```python
from build123d import *

# Parameters (mm, degrees)
F1_DEPTH = 3
F3_D     = 3
F5_D     = 3
F7_D     = 3
F9_D     = 16


with BuildPart() as f1:
    # F0 (on Top) → F1 (new body)
    with BuildSketch(Plane.XY):
        with BuildLine():
            Line((-25, 80.777472107), (-75, 80.777472107))
            ThreePointArc((-75, 80.777472107), (-120, 0), (-75, -80.777472107))
            Line((-75, -80.777472107), (-25, -80.777472107))
            ThreePointArc((-25, -80.777472107), (-70, 0), (-25, 80.777472107))
        make_face()
        with BuildLine():
            Line((25, 80.777472107), (-25, 80.777472107))
            ThreePointArc((-25, 80.777472107), (-70, 0), (-25, -80.777472107))
            Line((-25, -80.777472107), (25, -80.777472107))
            ThreePointArc((25, -80.777472107), (57.9909633635, -46.2331050223), (70, 0))
            ThreePointArc((70, 0), (57.9909633635, 46.2331050223), (25, 80.777472107))
        make_face()
        with BuildLine():
            Line((75, 80.777472107), (25, 80.777472107))
            ThreePointArc((25, 80.777472107), (57.9909633635, 46.2331050223), (70, 0))
            ThreePointArc((70, 0), (57.9909633635, -46.2331050223), (25, -80.777472107))
            Line((25, -80.777472107), (75, -80.777472107))
            ThreePointArc((75, -80.777472107), (107.9909633635, -46.2331050223), (120, 0))
            ThreePointArc((120, 0), (107.9909633635, 46.2331050223), (75, 80.777472107))
        make_face()
    extrude(amount=F1_DEPTH)

    # F3 (through all)
    with Locations(Plane.XY.offset(3)):
        with Locations((-50, 50), (50, 50), (50, -50), (-50, -50)):
            Hole(F3_D / 2)

    # F5 (through all)
    with Locations(Plane.XY.offset(3)):
        with Locations((-21.2132034356, 21.2132034356), (21.2132034356, 21.2132034356), (21.2132034356, -21.2132034356), (-21.2132034356, -21.2132034356)):
            Hole(F5_D / 2)

    # F7 (through all)
    with Locations(Plane(origin=(0, 0, 0), x_dir=(1, 0, 0), z_dir=(0, 0, -1))):
        with Locations((-24.5, 41.5), (24.5, 41.5), (24.5, -16.5), (-24.5, -16.5)):
            Hole(F7_D / 2)

    # F9 (through all)
    with Locations(Plane.XY.offset(3)):
        with Locations((-80, 0)):
            Hole(F9_D / 2)


solid = f1.part
```
Build history of the part. All positions in model axes, mm. Round coordinates to 2 decimals unless told otherwise and drop trailing zeros. Write each loop counter-clockwise with the first axis right and the second up, starting at its lowest first coordinate (ties: lowest second). Pieces come first, ordered by that corner, then holes. Notation, with made-up numbers: (72, 45.5) - (96, 45.5) arc R21 cw to (96, 79.5) - close; hole circle Ø5 at (-5, 74.5). An arc over 180 degrees is marked (long way). Answer as CSV lines item,"result".
Q1. Cut at B-B (z = 2.2). State how many separate pieces and enclosed holes the cut face has, and give its area (3 significant figures).
Report:
separate pieces,"1"
enclosed holes,"13"
area,"34,200 mm^2"
Q2. Pull direction Y, two halves, no side cores. Call faces 1 (the flat face through (-2, 1, 3)), 2 (the cylindrical face through (-119.99, 1.35, 1.48)), 3 (the cylindrical face through (-73.651, -4.868, 1.479)): +Y half, -Y half, draft (parallel to the pull), parting line (faces both ways), or undercut.
Report:
face 1,"draft"
face 2,"parting line"
face 3,"undercut"
Q3. Cut at D-D (y = 40.5). Write the cut outline in (x, z), and give its area (3 significant figures).
Report:
outline,"(-110.93, 0) - (110.93, 0) - (110.93, 3) - (-110.93, 3) - close"
area,"666 mm^2"
Q4. Drill centre lines: probe 1 along Y at (x, z) = (-24.5, 1.35); probe 2 along Y at (x, z) = (-50, 1.75); probe 3 along X at (y, z) = (16.5, 0.7). Where is each one in solid material? Low to high. Write a range as [from, to].
Report:
probe 1,"y = [-80.78, -43], [-40, 15], [18, 80.78]"
probe 2,"y = [-80.78, -51.5], [-48.5, 48.5], [51.5, 80.78]"
probe 3,"x = [-118.56, -26], [-23, 23], [26, 118.56]"
Q5. Cut at C-C (y = -59). Write the cut outline in (x, z), and give its area (3 significant figures).
Report:
outline,"(-99.46, 0) - (99.46, 0) - (99.46, 3) - (-99.46, 3) - close"
area,"597 mm^2"
Q6. Cut at A-A (x = -80). Write the cut outline in (y, z).
Report:
outline,"(-77.46, 0) - (-8, 0) - (-8, 3) - (-77.46, 3) - close; (8, 0) - (77.46, 0) - (77.46, 3) - (8, 3) - close"
